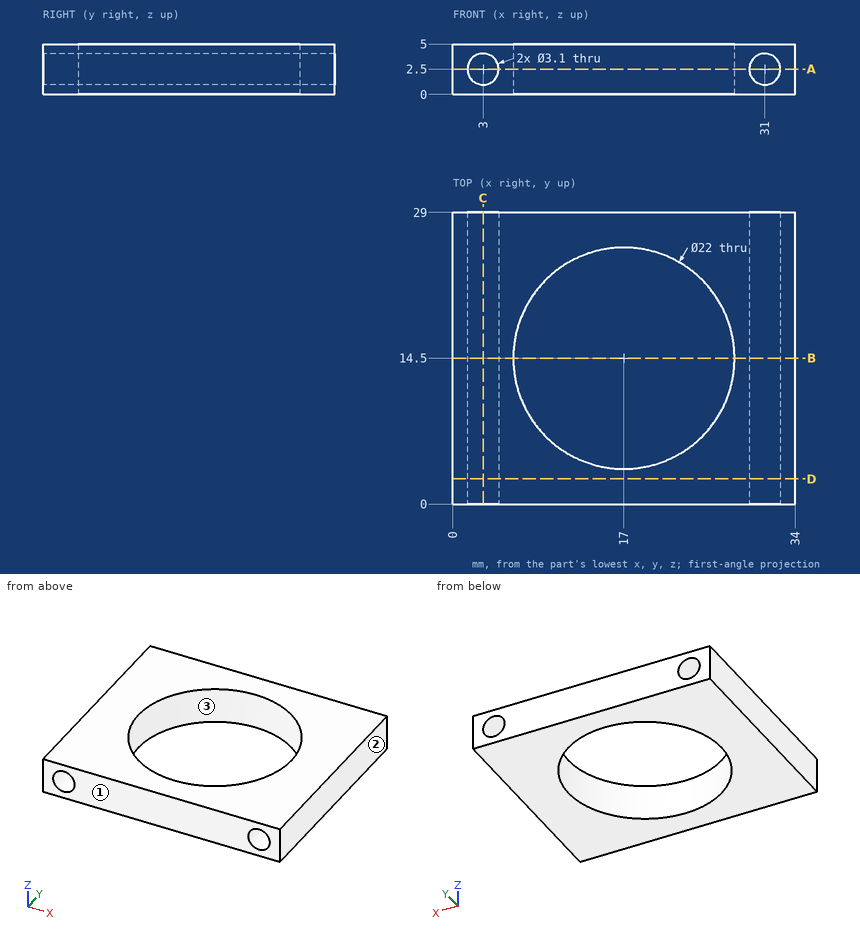
Source: three-view drawing plus pictorial views. Frame: mm from the lowest corner of the part. Give positions to 0.01 mm unless a question says otherwise; leave off trailing zeros. Loops run counter-clockwise (first coordinate to the right, second up) from the corner with the lowest first, then second, coordinate; pieces in that order, holes last. Notation, with made-up numbers: (3.25, -38) -> (33.25, -38) arc R32 ccw to (33.25, -12) -> close; hole circle Ø9 at (72, 56.25). An arc over 180 degrees is marked (long way). Put each result on its own line as item: value. Start each with the question number.
1) Contact query for a flat-ended pin moving along its axis: P1, Ø6, axis at x = 20.5, y = 10.5, coming from the +Z side. Output: stop coordinate, or through.
2) Draft query along X for the marked faces 1, 2 and 3. Return one class per face: released by +X, released by -X, zero draft, split by the parting line, or undercut.
3) Cut plane D-D (y = 2.5). Return loops of the section in (x, z), then the cut area to 3 significant figures.
4) Cut plane B-B (y = 14.5). Return loops of the section in (x, z).
5) Cut plane C-C (x = 3). Return loops of the section in (y, z), then the cut area to 3 significant figures.
6) Material intervals for probe 1 along Y at (x, z) = (17, 1.6); probe 2 along Z at (x, y) = (31, 18.5); probe 3 along X at (y, z) = (20.5, 1.8), sorted ascending.
7) Cut plane A-A (z = 2.5). Return loops of the section in (x, y).
Results are:
1. P1: passes through
2. face 1: zero draft
2. face 2: released by +X
2. face 3: undercut
3. outline: (0, 0) -> (34, 0) -> (34, 5) -> (0, 5) -> close; hole circle Ø3.1 at (3, 2.5); hole circle Ø3.1 at (31, 2.5)
3. area: 155 mm2
4. outline: (0, 0) -> (6, 0) -> (6, 5) -> (0, 5) -> close; (28, 0) -> (34, 0) -> (34, 5) -> (28, 5) -> close; hole circle Ø3.1 at (3, 2.5); hole circle Ø3.1 at (31, 2.5)
5. outline: (0, 0) -> (29, 0) -> (29, 0.95) -> (0, 0.95) -> close; (0, 4.05) -> (29, 4.05) -> (29, 5) -> (0, 5) -> close
5. area: 55.1 mm2
6. probe 1: y = 0 to 3.5, 25.5 to 29
6. probe 2: z = 0 to 0.95, 4.05 to 5
6. probe 3: x = 0 to 1.62, 4.38 to 7.78, 26.22 to 29.62, 32.38 to 34
7. outline: (0, 0) -> (1.45, 0) -> (1.45, 29) -> (0, 29) -> close; (4.55, 0) -> (29.45, 0) -> (29.45, 29) -> (4.55, 29) -> close; (32.55, 0) -> (34, 0) -> (34, 29) -> (32.55, 29) -> close; hole circle Ø22 at (17, 14.5)
